Check sheet for the modelled part. Datum: model origin and axes. Units: mm. Face numbers are marked on the shaded views. A direction names the side the tool comes from. Give positions to 0.01 mm unless a question says otherwise; leave off trailing zeros. Loops run counter-clockwise (first coordinate to the right, second up) from the corner with the lowest first, then second, coordinate; pieces in that order, holes last. Notation, with made-up numbers: (55.5, 55) - (75.5, 55) arc R24 cw to (75.5, 73) - close; hole circle Ø7 at (21, 14). An arc over 180 degrees is marked (long way). Use one line per item in the form item = value.
from build123d import *

# Parameters (mm, degrees)
SKETCH1_R           = 18
SKETCH1_R_2         = 10.75
BOSS_EXTRUDE1_DEPTH = 14
SKETCH2_R           = 3.25
BOSS_EXTRUDE2_DEPTH = 6
BOSS_EXTRUDE3_START = 24
SKETCH3_R           = 10
SKETCH3_R_2         = 3.25
BOSS_EXTRUDE3_DEPTH = 24


with BuildPart() as part:
    # Sketch1 → Boss-Extrude1 (new body)
    with BuildSketch(Plane.XY):
        Circle(SKETCH1_R)
        Circle(SKETCH1_R_2, mode=Mode.SUBTRACT)
    extrude(amount=BOSS_EXTRUDE1_DEPTH)

    # Sketch2 → Boss-Extrude2 (add)
    with BuildSketch(Plane(origin=(0, 0, 0), x_dir=(-1, 0, 0), z_dir=(0, 0, -1))):
        with BuildLine():
            ThreePointArc((40.105263158, -9.775881906), (48, 0), (40.105263158, 9.775881906))
            Line((40.105263158, 9.775881906), (3.789473684, 17.59658743))
            ThreePointArc((3.789473684, 17.59658743), (14.003758894, 11.309055524), (18, 0))
            ThreePointArc((18, 0), (14.003758894, -11.309055524), (3.789473684, -17.59658743))
            Line((3.789473684, -17.59658743), (40.105263158, -9.775881906))
        make_face()
        with Locations((38, 0)):
            Circle(SKETCH2_R, mode=Mode.SUBTRACT)
    extrude(amount=-BOSS_EXTRUDE2_DEPTH)

    # Sketch3 → Boss-Extrude3 (add)
    with BuildSketch(Plane(origin=(0, 0, 0), x_dir=(-1, 0, 0), z_dir=(0, 0, -1)).offset(BOSS_EXTRUDE3_START)):
        with Locations((38, 0)):
            Circle(SKETCH3_R)
        with Locations((38, 0)):
            Circle(SKETCH3_R_2, mode=Mode.SUBTRACT)
    extrude(amount=-BOSS_EXTRUDE3_DEPTH)


solid = part.part
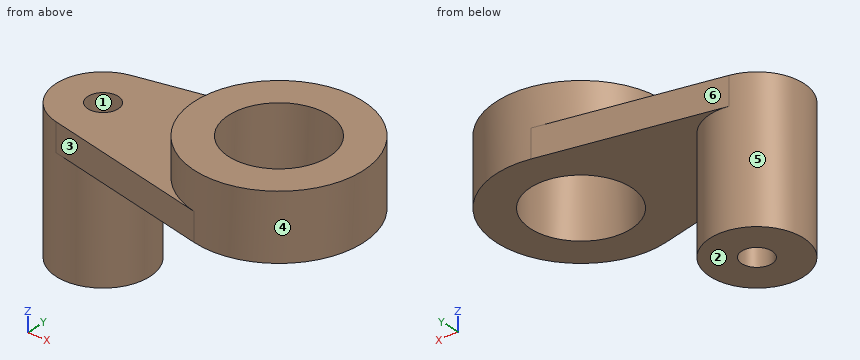
Item 1: Access from +Z, -Z, +X, -X, +Y, -Y to the whole of each face (thin tool, end or side, straight path). Record for the marked faces 4, 5 and 6.
Answer block:
face_4 = +Z
face_5 = -Z
face_6 = +Z, -Z, -X, +Y
Item 2: Mould release check, pull along Y, two halves, no side actions. Record for the marked faces 1, 2 and 3: released by +Y, released by -Y, zero draft, split by the parting line, or undercut.
Answer block:
face_1 = undercut
face_2 = zero draft
face_3 = released by -Y
Item 3: Section check B-B on y = 4. Record the boundary of the cut face in (x, z), then the cut area to 3 significant figures.
Answer block:
outline = (-47.17, -24) - (-28.83, -24) - (-28.83, 0) - (-9.98, 0) - (-9.98, 14) - (-17.55, 14) - (-17.55, 6) - (-47.17, 6) - close; (9.98, 0) - (17.55, 0) - (17.55, 14) - (9.98, 14) - close
area = 830 mm2
Item 4: Section check A-A on x = 0. Record the boundary of the cut face in (y, z), then the cut area to 3 significant figures.
Answer block:
outline = (-18, 0) - (-10.75, 0) - (-10.75, 14) - (-18, 14) - close; (10.75, 0) - (18, 0) - (18, 14) - (10.75, 14) - close
area = 203 mm2
Item 5: Section check D-D on z = -3. Record the boundary of the cut face in (x, y), then the cut area to 3 significant figures.
Answer block:
outline = circle Ø20 at (-38, 0); hole circle Ø6.5 at (-38, 0)
area = 281 mm2
Item 6: Section check C-C on z = 3.5. Record the boundary of the cut face in (x, y).
Answer block:
outline = (-40.11, -9.78) - (-3.79, -17.6) arc R18 ccw (long way) to (-3.79, 17.6) - (-40.11, 9.78) arc R10 ccw to start; hole circle Ø6.5 at (-38, 0); hole circle Ø21.5 at (0, 0)
Item 7: Gauge pin test, flat ends, axial feed: P1, Ø10, axis at x = 8, z = -8, coming from the +Y side; P2, Ø10, axis at y = 6, z = 4.5, coming from the +X side; P3, Ø12, axis at x = 7.5, y = -3, coming from the -Z side; P4, Ø10.5, axis at x = -29, y = 2, coming from the +Z side. Record the tip position at first contact, or that the pin passes through.
Answer block:
P1 = through
P2 = 17.97
P3 = 0
P4 = 6
Item 8: Thickness scan on L1, parallel to Y at x = -38, z = -7.5; L2, parallel to Y at x = 0, z = 10.5; L3, parallel to Z at x = -25.5, y = -11.5. Record the ranges inside material, lowest first.
Answer block:
L1 = -10 to -3.25, 3.25 to 10
L2 = -18 to -10.75, 10.75 to 18
L3 = 0 to 6
